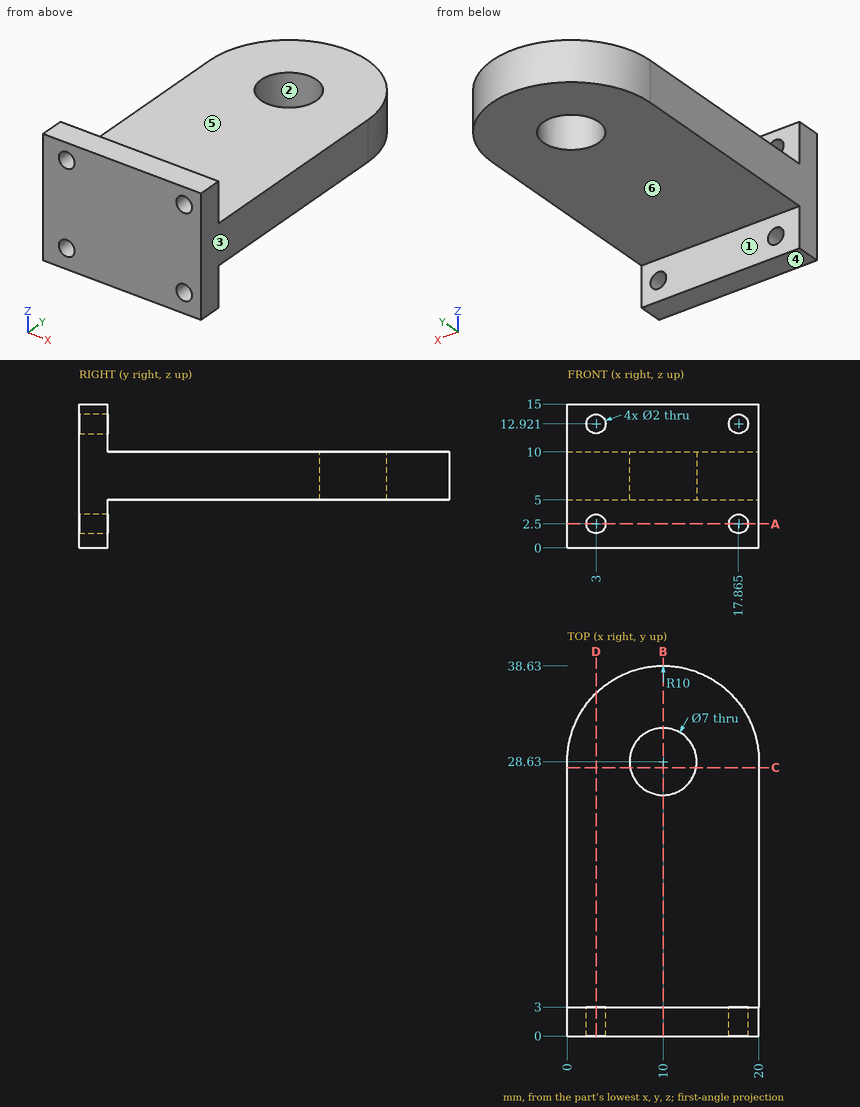
Study the drawing (mm; zero at the part's minimum x, y, z) and answer. A direction names the side the tool comes from. Round coordinates to 2 decimals unless told otherwise and drop trailing zeros. Write each loop counter-clockwise with the first axis right and the second up, starting at its lowest first coordinate (ties: lowest second). Pieces come first, ordered by that corner, then holes.
Q1. Find section A-A on z = 2.5. Determine the outline of the cut face in (x, y) (1 decimal).
Values:
outline: (0, 0) - (2, 0) - (2, 3) - (0, 3) - close; (4, 0) - (16.9, 0) - (16.9, 3) - (4, 3) - close; (18.9, 0) - (20, 0) - (20, 3) - (18.9, 3) - close
Q2. Find section B-B on x = 10. Determine the outline of the cut face in (y, z).
Values:
outline: (0, 0) - (3, 0) - (3, 5) - (25.13, 5) - (25.13, 10) - (3, 10) - (3, 15) - (0, 15) - close; (32.13, 5) - (38.63, 5) - (38.63, 10) - (32.13, 10) - close
Q3. Find section D-D on x = 3. Determine the outline of the cut face in (y, z), and give its area (3 significant figures).
Values:
outline: (0, 0) - (3, 0) - (3, 1.5) - (0, 1.5) - close; (0, 3.5) - (3, 3.5) - (3, 5) - (35.77, 5) - (35.77, 10) - (3, 10) - (3, 11.92) - (0, 11.92) - close; (0, 13.92) - (3, 13.92) - (3, 15) - (0, 15) - close
area: 197 mm2
Q4. Flat-ended cylindrical pins translate along their axes: P1, Ø3, axis at x = 3, y = 12, coming from the +Z side; P2, Ø1, axis at x = 6.5, z = 6, coming from the +Y side; P3, Ø5.5, axis at x = 6, z = 13.5, coming from the +Y side; P4, Ø1.6, axis at x = 17.87, z = 2.5, coming from the +Y side. Find the tip coordinate at first contact, or state that the pin passes through.
Values:
P1: stops at z = 10
P2: stops at y = 38.17
P3: stops at y = 3
P4: passes through
Q5. The mould has two halves that part along X. Classify the marked faces 1, 2 and 3: released by +X, released by -X, zero draft, split by the parting line, or undercut.
Values:
face 1: zero draft
face 2: undercut
face 3: released by +X
Q6. A tool of negligible diameter and unlimited length cuts with its end or side. For the marked faces 4, 5 and 6, from which of +Z, -Z, +X, -X, +Y, -Y can it reach the whole face along a straight path? Write none if from no direction.
Values:
face 4: -Z, +X, -X, +Y, -Y
face 5: +Z, +X, -X, +Y
face 6: -Z, +X, -X, +Y
Q7. Find section C-C on y = 28. Determine the outline of the cut face in (x, z).
Values:
outline: (0, 5) - (6.56, 5) - (6.56, 10) - (0, 10) - close; (13.44, 5) - (20, 5) - (20, 10) - (13.44, 10) - close
Q8. Straight lines are drawn through the part: line 1 (X direction, y = 1.75, z = 2.5) (1 decimal); line 2 (Y direction, x = 13.5, z = 11.75); line 3 (Y direction, x = 10, z = 8.65). For each, find the intervals that lie inside material, in ascending order.
Values:
line 1: x = 0 to 2, 4 to 16.9, 18.9 to 20
line 2: y = 0 to 3
line 3: y = 0 to 25.13, 32.13 to 38.63
